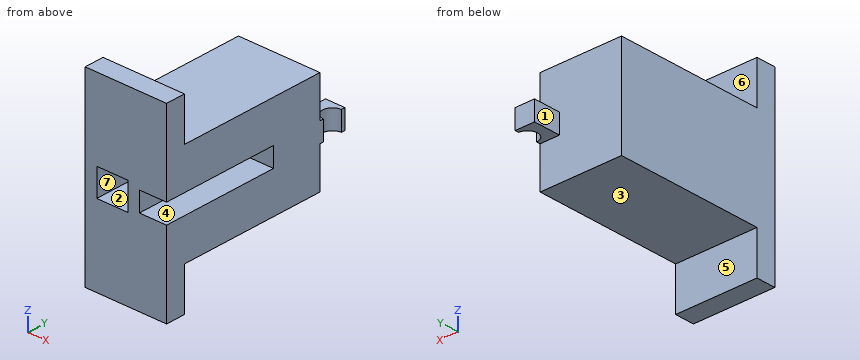
from build123d import *

# Parameters (mm, degrees)
EXTRUDE_1_DEPTH          = 50
SKETCH_3_W               = 8
SKETCH_3_H               = 7
CUT_EXTRUDE_1_DEPTH      = 31.389642439
CUT_EXTRUDE_2_DEPTH      = 55.893077888
CUT_EXTRUDE_2_DEPTH_BACK = 30
SKETCH_15_W              = 6
SKETCH_15_H              = 7
CUT_EXTRUDE_10_DEPTH     = 30
SKETCH_16_W              = 16
SKETCH_16_H              = 7
SKETCH_16_W_2            = 6.921662606
CUT_EXTRUDE_11_DEPTH     = 30
SKETCH_18_R              = 2.5
CUT_EXTRUDE_12_DEPTH     = 30
SKETCH_19_W              = 21
SKETCH_19_H              = 3
CUT_EXTRUDE_14_DEPTH     = 50
SKETCH_20_W              = 4
SKETCH_20_H              = 6.019641958
CUT_EXTRUDE_16_DEPTH     = 50
EXTRUDE_START            = -43
SKETCH_21_W              = 21
SKETCH_21_H              = 7.5
EXTRUDE_3_DEPTH          = 43
SKETCH_22_W              = 21
SKETCH_22_H              = 5
EXTRUDE_4_DEPTH          = 11
SKETCH_23_W              = 21
SKETCH_23_H              = 5
EXTRUDE_5_DEPTH          = 11


with BuildPart() as part:
    # 草图1 → 凸台-拉伸1 (new body)
    with BuildSketch(Plane(origin=(0, 0, 0), x_dir=(1, 0, 0), z_dir=(0, 1, 0))):
        Polygon((0, -8.5), (0, -1), (-2, -1), (-2, -3), (-4, -3), (-4, 3), (-2, 3), (-2, 1), (0, 1), (0, 8.5), (21, 8.5), (21, -8.5), align=None)
    extrude(amount=EXTRUDE_1_DEPTH)

    # 草图3 → 切除-拉伸1 (cut)
    with BuildSketch(Plane.XZ):
        with Locations((7, 0)):
            Rectangle(SKETCH_3_W, SKETCH_3_H)
    extrude(amount=-CUT_EXTRUDE_1_DEPTH, mode=Mode.SUBTRACT)

    # 草图6 → 切除-拉伸2 (cut, two sides: drawn at the far end of the back side and taken through both)
    with BuildSketch(Plane.XZ.offset(-CUT_EXTRUDE_2_DEPTH_BACK)):
        Polygon((21, -2.405859061), (21, 0), (21, 2.5), (14, 2.5), (14, -2.5), (21, -2.5), align=None)
    extrude(amount=CUT_EXTRUDE_2_DEPTH + CUT_EXTRUDE_2_DEPTH_BACK, mode=Mode.SUBTRACT)

    # 草图15 → 切除-拉伸10 (cut)
    with BuildSketch(Plane(origin=(21, 0, 0), x_dir=(0, 0, -1), z_dir=(1, 0, 0))):
        with Locations((-5.5, 46.5)):
            Rectangle(SKETCH_15_W, SKETCH_15_H)
        with Locations((5.5, 46.5)):
            Rectangle(SKETCH_15_W, SKETCH_15_H)
    extrude(amount=-CUT_EXTRUDE_10_DEPTH, mode=Mode.SUBTRACT)

    # 草图16 → 切除-拉伸11 (cut)
    with BuildSketch(Plane.XY.offset(2.5)):
        with Locations((8, 46.5)):
            Rectangle(SKETCH_16_W, SKETCH_16_H)
        with Locations((-3.460831303, 46.5)):
            Rectangle(SKETCH_16_W_2, SKETCH_16_H)
    extrude(amount=-CUT_EXTRUDE_11_DEPTH, mode=Mode.SUBTRACT)

    # 草图18 → 切除-拉伸12 (cut)
    with BuildSketch(Plane(origin=(0, 0, -2.5), x_dir=(-1, 0, 0), z_dir=(0, 0, -1))):
        with Locations((-21, 46.5)):
            Circle(SKETCH_18_R)
    extrude(amount=-CUT_EXTRUDE_12_DEPTH, mode=Mode.SUBTRACT)

    # 草图19 → 切除-拉伸14 (cut)
    with BuildSketch(Plane(origin=(0, 0, 0), x_dir=(-1, 0, 0), z_dir=(0, -1, 0))):
        with Locations((-10.5, -7)):
            Rectangle(SKETCH_19_W, SKETCH_19_H)
        with Locations((-10.5, 7)):
            Rectangle(SKETCH_19_W, SKETCH_19_H)
    extrude(amount=-CUT_EXTRUDE_14_DEPTH, mode=Mode.SUBTRACT)

    # 草图20 → 切除-拉伸16 (cut)
    with BuildSketch(Plane.XZ):
        with Locations((-2, -0.009820979)):
            Rectangle(SKETCH_20_W, SKETCH_20_H)
    extrude(amount=-CUT_EXTRUDE_16_DEPTH, mode=Mode.SUBTRACT)

    # 草图21 → 凸台-拉伸3 (add)
    with BuildSketch(Plane.XZ.offset(EXTRUDE_START)):
        with Locations((10.5, -9.25)):
            Rectangle(SKETCH_21_W, SKETCH_21_H)
        with Locations((10.5, 9.25)):
            Rectangle(SKETCH_21_W, SKETCH_21_H)
    extrude(amount=EXTRUDE_3_DEPTH)

    # 草图22 → 凸台-拉伸4 (add)
    with BuildSketch(Plane.XY.offset(13)):
        with Locations((10.5, 2.5)):
            Rectangle(SKETCH_22_W, SKETCH_22_H)
    extrude(amount=EXTRUDE_4_DEPTH)

    # 草图23 → 凸台-拉伸5 (add)
    with BuildSketch(Plane(origin=(0, 0, -13), x_dir=(-1, 0, 0), z_dir=(0, 0, -1))):
        with Locations((-10.5, 2.5)):
            Rectangle(SKETCH_23_W, SKETCH_23_H)
    extrude(amount=EXTRUDE_5_DEPTH)


solid = part.part
Input: part model. Units: mm. Frame: model coordinates. Face numbers are marked on the shaded views. A direction names the side the tool comes from. Give positions to 0.01 mm unless a question says otherwise; leave off trailing zeros. Order: outer loops, then holes, each group sorted by start corner. A loop starts at its lowest first (then second) coordinate and runs counter-clockwise, first axis right, second up. Notation, with made-up numbers: M 24.5,27 L 75.5,27 A13 cw 75.5,38 Z; hole C -17,9.25 d7. An arc over 180 degrees is marked long. Answer as a JSON object with one key per item and string values.
1. Cut plane D-D, the plane z = -21. Output: boundary loops of the cut face in (x, y), and give its area (3 significant figures).
Result sheet:
{"outline": "M 0,0 L 21,0 L 21,5 L 0,5 Z", "area": "105 mm²"}
2. Pull-direction query (Z, two-part tool) for the marked faces 1, 2 and 3; classes: +Z half, -Z half, draft (parallel to the pull), parting line (faces both ways), or undercut.
Result sheet:
{"face 1": "draft", "face 2": "undercut", "face 3": "-Z half"}
3. Cut plane A-A, the plane y = 3.5. Output: boundary loops of the cut face in (x, z), and give its area (3 significant figures).
Result sheet:
{"outline": "M 0,-24 L 21,-24 L 21,-2.5 L 14,-2.5 L 14,2.5 L 21,2.5 L 21,24 L 0,24 Z; hole M 3,-3.5 L 11,-3.5 L 11,3.5 L 3,3.5 Z", "area": "917 mm²"}
4. Cut plane C-C, the plane y = 14.5. Output: boundary loops of the cut face in (x, z), and give its area (3 significant figures).
Result sheet:
{"outline": "M 0,-13 L 21,-13 L 21,-2.5 L 14,-2.5 L 14,2.5 L 21,2.5 L 21,13 L 0,13 Z; hole M 3,-3.5 L 11,-3.5 L 11,3.5 L 3,3.5 Z", "area": "455 mm²"}
5. Reachability of the marked faces 4, 5, 6 and 7 from +Z, -Z, +X, -X, +Y, -Y: full face, straight path, thin tool, end or side. Return the list, or none.
Result sheet:
{"face 4": "+X, -Y", "face 5": "-Z, +X, -X, +Y", "face 6": "+Z, +X, -X, +Y", "face 7": "-Y"}
6. Cut plane B-B, the plane x = 6. Output: boundary loops of the cut face in (y, z).
Result sheet:
{"outline": "M 0,-24 L 5,-24 L 5,-13 L 43,-13 L 43,13 L 5,13 L 5,24 L 0,24 L 0,3.5 L 31.39,3.5 L 31.39,-3.5 L 0,-3.5 Z"}
7. First-contact query: P1, Ø4, axis at x = 5, z = 19, coming from the -Y side; P2, Ø5.5, axis at x = 19, y = 45.5, coming from the +Z side; P3, Ø3.5, axis at x = 12.5, z = 19.5, coming from the +Y side; P4, Ø2, axis at x = 8, z = 1.5, coming from the -Y side. Flat tips, straight axial feed; report the tip coordinate or a pass-through.
Result sheet:
{"P1": "y = 0", "P2": "z = 13", "P3": "y = 5", "P4": "y = 31.39"}
8. Ray query, line 1 (Z direction, x = 9.5, y = 24); line 2 (Z direction, x = 14.75, y = 2); line 3 (Z direction, x = 1, y = 38.5). Return the intervals inside material, ascending. Write a range as [from, to].
Result sheet:
{"line 1": "[-13, -3.5], [3.5, 13]", "line 2": "[-24, -2.5], [2.5, 24]", "line 3": "[-13, 13]"}
